Geometry check sheet. Reference: the model listing, model coordinates, mm. A direction names the side the tool comes from. Coordinates: 2 decimals unless noted, no trailing zeros. Write each loop counter-clockwise with the first axis right and the second up, starting at its lowest first coordinate (ties: lowest second). Pieces come first, ordered by that corner, then holes. Notation, with made-up numbers: (11, -37) -> (40, -37) arc R19 ccw to (40, -8) -> close; hole circle Ø7 at (77.25, -13.5). An arc over 180 degrees is marked (long way). Answer in a Markdown table with one row per item. Add a question column.
1. Depth check by flat-ended pin: P1, Ø2.5, axis at x = 8, z = 20, coming from the -Y side; P2, Ø8, axis at y = 3.5, z = -13.5, coming from the -X side; P3, Ø3, axis at x = -12, z = 2.5, coming from the +Y side; P4, Ø3, axis at y = 3.5, z = -15, coming from the +X side. Enter the tip coordinate at first touch or a pass-through.
2. Mould release check, pull along Y, two halves, no side actions. Record for faces 1 (the flat face through (-6, 4, -15)), 2 (the cylindrical face through (17.46, 40.65, 0.89)), 3 (the flat face through (17, 6, 8)): pulls with the +Y half, pulls with the -Y half, needs draft (parallel to the pull), parting line crosses it, or undercut.
3. Cross-section at B-B on z = 20. Record the cut outline in (x, y).
4. Cross-section at C-C on x = 8. Record the cut outline in (y, z).
5. Cross-section at D-D on x = -7. Record the cut outline in (y, z), and give its area (3 significant figures).
6. Set-up check for faces 4 (the flat face through (17, 24, 7)), 5 (the flat face through (-16, 4, -15)), 6 (the flat face through (-21, 4, -15)): record each of +Z, -Z, +X, -X, +Y, -Y from which the full face is reachable in a straight line by a thin tool's end or side.
7. Cross-section at A-A on x = -20. Record the cut outline in (y, z).
8. Scan lines: L1, parallel to X at y = 3, z = 0; L2, parallel to X at y = 5, z = -14.5; L3, parallel to Z at x = 8, y = 2.15. Record each from-to range of solid material in increasing order. Write a range as from..to.
```python
from build123d import *

# Parameters (mm, degrees)
SKETCH_1_W                 = 50
SKETCH_1_H                 = 43
EXTRUDE_1_DEPTH            = 5
EXTRUDE_2_DEPTH            = 5
EXTRUDE_START              = -6
EXTRUDE_3_DEPTH            = 5
EXTRUDE_START_2            = 5
SKETCH_6_R                 = 5
EXTRUDE_4_DEPTH            = 5
SKETCH_7_W                 = 5
SKETCH_7_H                 = 11
SKETCH_7_W_2               = 21
SKETCH_7_W_3               = 4
CUT_EXTRUDE_1_DEPTH        = 54.116947969
CUT_EXTRUDE_2_DEPTH        = 69.138244203
CUT_EXTRUDE_2_DEPTH_BACK   = 69.138244203
SKETCH_9_R                 = 1.5
CHAMFER_1_SIZE             = 2
SKETCH_10_R                = 1.5
CUT_EXTRUDE_3_DEPTH        = 65.944748233
RIB_1_REACH                = 70.138
SKETCH_11_WALL_W           = 172.917504556
SKETCH_11_WALL_H           = 5
CHAMFER_2_SIZE             = 2
HOLE_WIZARD_M3_1_OUTLINE_R = 1.5
HOLE_WIZARD_M3_1_DEPTH     = 5


# Read off the part's stored shape, not the designer's step: M3 螺纹孔1
with BuildPart() as part:
    # 草图1 → 凸台-拉伸1 (new body)
    with BuildSketch(Plane(origin=(0, 0, 0), x_dir=(1, 0, 0), z_dir=(0, 1, 0))):
        with Locations((0, -3.5)):
            Rectangle(SKETCH_1_W, SKETCH_1_H)
    extrude(amount=EXTRUDE_1_DEPTH)

    # 草图3 → 凸台-拉伸2 (add)
    with BuildSketch(Plane(origin=(20, 0, 0), x_dir=(0, 0, -1), z_dir=(1, 0, 0))):
        with BuildLine():
            Line((13.669872981, 2.5), (-6.330127019, 37.141016151))
            ThreePointArc((-6.330127019, 37.141016151), (-4.5, 43.97114317), (2.330127019, 42.141016151))
            Line((2.330127019, 42.141016151), (22.330127019, 7.5))
            ThreePointArc((22.330127019, 7.5), (20.5, 0.669872981), (13.669872981, 2.5))
        make_face()
    extrude(amount=-EXTRUDE_2_DEPTH)

    # 草图5 → 凸台-拉伸3 (add)
    with BuildSketch(Plane(origin=(0, 0, 0), x_dir=(0, 0, -1), z_dir=(1, 0, 0)).offset(EXTRUDE_START)):
        with BuildLine():
            ThreePointArc((22.330127019, 7.5), (13.669872981, 7.5), (18, 0))
            ThreePointArc((18, 0), (21.535533906, 1.464466094), (23, 5))
            ThreePointArc((23, 5), (22.829629131, 6.294095226), (22.330127019, 7.5))
        make_face()
    extrude(amount=-EXTRUDE_3_DEPTH)

    # 草图6 → 凸台-拉伸4 (add)
    with BuildSketch(Plane(origin=(-21, 0, 0), x_dir=(0, 0, -1), z_dir=(1, 0, 0)).offset(EXTRUDE_START_2)):
        with Locations((18, 5)):
            Circle(SKETCH_6_R)
    extrude(amount=-EXTRUDE_4_DEPTH)

    # 草图7 → 切除-拉伸1 (cut, through all)
    with BuildSketch(Plane(origin=(0, 5, 0), x_dir=(1, 0, 0), z_dir=(0, 1, 0))):
        with Locations((-13.5, 12.5)):
            Rectangle(SKETCH_7_W, SKETCH_7_H)
        with Locations((4.5, 12.5)):
            Rectangle(SKETCH_7_W_2, SKETCH_7_H)
        with Locations((22.5, 12.5)):
            Rectangle(SKETCH_7_W, SKETCH_7_H)
        with Locations((-23, 12.5)):
            Rectangle(SKETCH_7_W_3, SKETCH_7_H)
    extrude(amount=-CUT_EXTRUDE_1_DEPTH, mode=Mode.SUBTRACT)

    # 草图9 → 切除-拉伸2 (cut, two sides: drawn at the far end of the back side and taken through both)
    with BuildSketch(Plane(origin=(20, 0, 0), x_dir=(0, 0, -1), z_dir=(1, 0, 0)).offset(-CUT_EXTRUDE_2_DEPTH_BACK)):
        with Locations((18, 5)):
            Circle(SKETCH_9_R)
    extrude(amount=CUT_EXTRUDE_2_DEPTH + CUT_EXTRUDE_2_DEPTH_BACK, mode=Mode.SUBTRACT)

    # 倒角1
    chamfer_1_edges = [part.edges().sort_by_distance(p)[0] for p in [
        (-25, 2.5, -7),
        (25, 2.5, 25),
        (25, 2.5, -7),
        (-25, 2.5, 25),
    ]]
    chamfer(chamfer_1_edges, length=CHAMFER_1_SIZE)

    # 草图10 → 切除-拉伸3 (cut, through all)
    with BuildSketch(Plane.ZY.offset(-15)):
        with Locations((2, 39.641016151)):
            Circle(SKETCH_10_R)
    extrude(amount=-CUT_EXTRUDE_3_DEPTH, mode=Mode.SUBTRACT)

    # 草图11 wall → 筋1 (add, up to next)
    with BuildSketch(Plane(origin=(20, 22.320508076, 7), x_dir=(0, -1, 0), z_dir=(0, 0, -1)), mode=Mode.PRIVATE) as rib_1_sk1:
        with Locations((0, 2.5)):
            Rectangle(SKETCH_11_WALL_W, SKETCH_11_WALL_H)
    rib_1_tool1 = extrude(rib_1_sk1.sketch, amount=RIB_1_REACH, mode=Mode.PRIVATE) - part.part
    add(rib_1_tool1.solids().sort_by_distance((20, 22.320508076, 7))[0])

    # 倒角2
    chamfer_2_edges = [part.edges().sort_by_distance(p)[0] for p in [
        (15, 5, 0),
        (17.5, 5, 7),
        (20, 5, 0),
        (20, 2.5, -7),
        (15, 2.5, -7),
    ]]
    chamfer(chamfer_2_edges, length=CHAMFER_2_SIZE)

    # M3 螺纹孔1 outline → M3 螺纹孔1 (cut)
    with BuildSketch(Plane(origin=(0, 0, 0), x_dir=(1, 0, 0), z_dir=(0, 1, 0))):
        with Locations((8, 0)):
            Circle(HOLE_WIZARD_M3_1_OUTLINE_R)
        with Locations((-20, -20)):
            Circle(HOLE_WIZARD_M3_1_OUTLINE_R)
        with Locations((-20, 0)):
            Circle(HOLE_WIZARD_M3_1_OUTLINE_R)
        with Locations((8, -20)):
            Circle(HOLE_WIZARD_M3_1_OUTLINE_R)
    extrude(amount=HOLE_WIZARD_M3_1_DEPTH, mode=Mode.SUBTRACT)


solid = part.part
```
Results found:
| question | item | result |
|---|---|---|
| 1 | P1 | passes through |
| 1 | P2 | stops at x = -21 |
| 1 | P3 | stops at y = 5 |
| 1 | P4 | stops at x = 20 |
| 2 | face 1 | needs draft |
| 2 | face 2 | undercut |
| 2 | face 3 | pulls with the +Y half |
| 3 | outline | (-25, 0) -> (-21.5, 0) -> (-21.5, 5) -> (-25, 5) -> close; (-18.5, 0) -> (6.5, 0) -> (6.5, 5) -> (-18.5, 5) -> close; (9.5, 0) -> (25, 0) -> (25, 5) -> (9.5, 5) -> close |
| 4 | outline | (0, -7) -> (5, -7) -> (5, -1.5) -> (0, -1.5) -> close; (0, 1.5) -> (5, 1.5) -> (5, 18.5) -> (0, 18.5) -> close; (0, 21.5) -> (5, 21.5) -> (5, 25) -> (0, 25) -> close |
| 5 | outline | (0, -18) arc R5 ccw (long way) to (5, -13) -> (5, 25) -> (0, 25) -> close; hole circle Ø3 at (5, -18) |
| 5 | area | 267 mm^2 |
| 6 | face 4 | +Z, +X, -X, +Y |
| 6 | face 5 | -Z, +Y, -Y |
| 6 | face 6 | -Z, -X, +Y, -Y |
| 7 | outline | (0, -18) arc R5 ccw (long way) to (5, -13) -> (5, -1.5) -> (0, -1.5) -> close; (0, 1.5) -> (5, 1.5) -> (5, 18.5) -> (0, 18.5) -> close; (0, 21.5) -> (5, 21.5) -> (5, 25) -> (0, 25) -> close; hole circle Ø3 at (5, -18) |
| 8 | L1 | x = -25..-21.5, -18.5..6.5, 9.5..25 |
| 8 | L2 | x = -21..-16, -11..-6, 15..20 |
| 8 | L3 | z = -7..-1.5, 1.5..18.5, 21.5..25 |
